The model under review builds one solid part; all positions refer to its coordinate system, in mm. Round coordinates to 2 decimals unless told otherwise and drop trailing zeros. Loops run counter-clockwise (first coordinate to the right, second up) from the corner with the lowest first, then second, coordinate; pieces in that order, holes last. Notation, with made-up numbers: (16, 22) - (29, 22) arc R13 ccw to (29, 42) - close; hole circle Ø11 at (2, 50.5). An arc over 180 degrees is marked (long way). Answer as CSV lines item,"result".
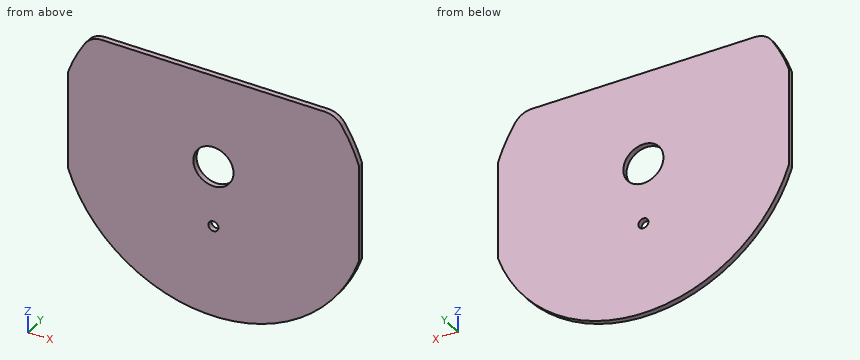
Autodesk Inventor part; units mm, degrees
ref_plane "YZ Plane" through (0, 0, 0) normal (1, 0, 0) x (0, 1, 0)
ref_plane "XZ Plane" through (0, 0, 0) normal (0, 1, 0) x (-1, 0, 0)
ref_plane "XY Plane" through (0, 0, 0) normal (0, 0, 1) x (1, 0, 0)
sketch "Sketch3" plane through (0, 0, 0) normal (0, 1, 0) x (-1, 0, 0)
  line L0 (0, 0) -> (72.5, 0)
  line L1 (0, 0) -> (0, 46.5)
  line L2 (72.5, 24.4131) -> (72.5, -24.4131)
  line L3 (0, 46.5) -> (55.5878, 46.5)
  line L4 (-72.5, 24.4131) -> (-72.5, -24.4131)
  line L5 (0, 46.5) -> (-55.5878, 46.5)
  arc A0 (72.5, 24.4131) -> (63.9468, 41.9887) centre (0, 0) ccw
  arc A1 (-63.9468, 41.9887) -> (-72.5, 24.4131) centre (0, 0) ccw
  arc A2 (-72.5, -24.4131) -> (72.5, -24.4131) centre (0, 0) ccw
  arc A3 (63.9468, 41.9887) -> (55.5878, 46.5) centre (55.5878, 36.5) ccw
  arc A4 (-55.5878, 46.5) -> (-63.9468, 41.9887) centre (-55.5878, 36.5) ccw
  point P0 (60.7454, 46.5)
  point P1 (-60.7454, 46.5)
  dimension "d28" = 72.5
  dimension "d29" = 46.5
  dimension "d30" = 10
  dimension "d31" = 10
  dimension "d32" = 76.5
  dimension "d34" = 72.5
  dimension "d35" = 76.5
extrude "Extrusion2" add sketch "Sketch3" along normal blind 2.7
sketch "Sketch4" plane through (0, 2.7, 0) normal (0, 1, 0) x (1, 0, 0)
  line L0 (-55.5878, -46.5) -> (55.5878, -46.5)
  line L1 (0, -46.5) -> (0, 0)
  circle A0 centre (0, 0) radius 10
  arc A1 (72.5, 24.4131) -> (-72.5, 24.4131) centre (0, 0) ccw
  line L2 (0, 76.5) -> (0, 30.5)
  circle A2 centre (0, 30.5) radius 2.5
  dimension "d36" = 20
  dimension "d37" = 46
  dimension "d38" = 5
extrude "Extrusion3" cut sketch "Sketch4" against normal blind 10
properties part number "tapa_carcasa_4.0"
1. Take a section at D-D (z = -30.5). State the section outline as (x, y) points.
Numbers:
outline,"(-70.16, 0) - (-2.5, 0) - (-2.5, 2.7) - (-70.16, 2.7) - close; (2.5, 0) - (70.16, 0) - (70.16, 2.7) - (2.5, 2.7) - close"
2. Take a section at A-A (z = 0). State the section outline as (x, y) points, plus the area to 4 significant figures.
Numbers:
outline,"(-72.5, 0) - (-10, 0) - (-10, 2.7) - (-72.5, 2.7) - close; (10, 0) - (72.5, 0) - (72.5, 2.7) - (10, 2.7) - close"
area,"337.5 mm²"
3. Take a section at B-B (x = 0). State the section outline as (y, z) points, plus the area to 3 significant figures.
Numbers:
outline,"(0, -76.5) - (2.7, -76.5) - (2.7, -33) - (0, -33) - close; (0, -28) - (2.7, -28) - (2.7, -10) - (0, -10) - close; (0, 10) - (2.7, 10) - (2.7, 46.5) - (0, 46.5) - close"
area,"265 mm²"
4. Wall thickness on probe 1 along X at (y, z) = (0.7, 0); probe 2 along X at (y, z) = (2.3, -5.5); probe 3 along Z at (x, y) = (36.5, 1.7): over which ranges is each line inside the solid? List them lowest first.
Numbers:
probe 1,"x = -72.5 to -10, 10 to 72.5"
probe 2,"x = -72.5 to -8.35, 8.35 to 72.5"
probe 3,"z = -67.23 to 46.5"
5. Take a section at C-C (y = 0.6). State the section outline as (x, z) points, plus the area to 3 significant figures.
Numbers:
outline,"(-72.5, -24.41) arc R76.5 ccw to (72.5, -24.41) - (72.5, 24.41) arc R76.5 ccw to (63.95, 41.99) arc R10 ccw to (55.59, 46.5) - (-55.59, 46.5) arc R10 ccw to (-63.95, 41.99) arc R76.5 ccw to (-72.5, 24.41) - close; hole circle Ø20 at (0, 0); hole circle Ø5 at (0, -30.5)"
area,"15,200 mm²"
